```python
from build123d import *

# Parameters (mm, degrees)
F0_W          = 40
F0_H          = 25
F1_DEPTH      = 45
F2_R          = 5
F3_DEPTH      = 7
F4_R          = 2.5
F5_DEPTH      = 45.001
F5_DEPTH_BACK = 7.001
F6_R          = 2.5
F7_DEPTH      = 25.001


with BuildPart() as f1:
    # F0 (on Front) → F1 (new body)
    with BuildSketch(Plane.XZ):
        with Locations((-10, 0)):
            Rectangle(F0_W, F0_H)
    extrude(amount=-F1_DEPTH)

    # F2 (on face) → F3 (join)
    with BuildSketch(Plane.XZ):
        Circle(F2_R)
    extrude(amount=F3_DEPTH)

    # F4 (on Front) → F5 (cut, two sides)
    with BuildSketch(Plane.XZ) as f5_sk:
        Circle(F4_R)
    extrude(amount=-F5_DEPTH, mode=Mode.SUBTRACT)
    extrude(f5_sk.sketch, amount=F5_DEPTH_BACK, mode=Mode.SUBTRACT)

    # F6 (on face) → F7 (cut, through all)
    with BuildSketch(Plane.XY.offset(12.5)):
        with Locations((0, 21)):
            Circle(F6_R)
        with Locations((-10, 31)):
            Circle(F6_R)
        with Locations((-20, 21)):
            Circle(F6_R)
    extrude(amount=-F7_DEPTH, mode=Mode.SUBTRACT)


solid = f1.part
```
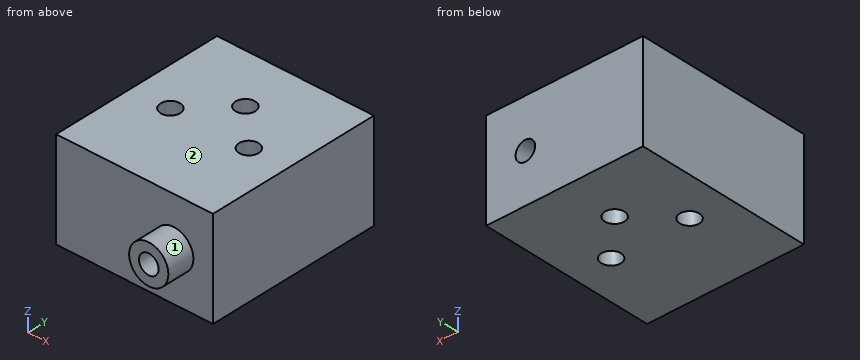
Geometry: final body of the model. Coordinates: model frame, mm. Face numbers are marked on the shaded views. A direction names the side the tool comes from. Coordinates: 2 decimals unless noted, no trailing zeros. Order: outer loops, then holes, each group sorted by start corner. A loop starts at its lowest first (then second) coordinate and runs counter-clockwise, first axis right, second up.
Item 1: Section query C-C (x = -10). Output: boundary loops of the cut face in (y, z), then the cut area to 3 significant figures.
Answer:
outline: (0, -12.5) - (28.5, -12.5) - (28.5, 12.5) - (0, 12.5) - close; (33.5, -12.5) - (45, -12.5) - (45, 12.5) - (33.5, 12.5) - close
area: 1,000 mm2
Item 2: Section query D-D (y = -1). Output: boundary loops of the cut face in (x, z), then the cut area to 3 significant figures.
Answer:
outline: circle Ø10 at (0, 0); hole circle Ø5 at (0, 0)
area: 58.9 mm2
Item 3: Section query A-A (x = 0). Output: boundary loops of the cut face in (y, z).
Answer:
outline: (-7, -5) - (0, -5) - (0, -12.5) - (18.5, -12.5) - (18.5, -2.5) - (-7, -2.5) - close; (-7, 2.5) - (18.5, 2.5) - (18.5, 12.5) - (0, 12.5) - (0, 5) - (-7, 5) - close; (23.5, -12.5) - (45, -12.5) - (45, -2.5) - (23.5, -2.5) - close; (23.5, 2.5) - (45, 2.5) - (45, 12.5) - (23.5, 12.5) - close
Item 4: Material intervals for line 1 along Y through (x, z) = (0, 4.75); line 2 along X through (y, z) = (14.5, 0); line 3 along Y through (x, z) = (-24, -9), sorted ascending.
Answer:
line 1: y = -7 to 18.5, 23.5 to 45
line 2: x = -30 to -2.5, 2.5 to 10
line 3: y = 0 to 45
Item 5: Section query B-B (z = 8). Output: boundary loops of the cut face in (x, y), then the cut area to 3 significant figures.
Answer:
outline: (-30, 0) - (10, 0) - (10, 45) - (-30, 45) - close; hole circle Ø5 at (-20, 21); hole circle Ø5 at (-10, 31); hole circle Ø5 at (0, 21)
area: 1,740 mm2
Item 6: Contact query for flat-ended pins moving along their axis: P1, Ø4, axis at x = 0, y = 21, coming from the +Z side; P2, Ø1.5, axis at x = -18.5, z = 0, coming from the -Y side; P3, Ø8, axis at x = -20, y = 21, coming from the +Z side. Output: stop coordinate, or through.
Answer:
P1: passes through
P2: stops at y = 0
P3: stops at z = 12.5
Item 7: Access query for the marked faces 1 and 2. Directions: +Z, -Z, +X, -X, +Y, -Y. A direction counts if a zero-diameter tool reaches every point of the face in a straight line with its end or side. Return the directions, or none.
Answer:
face 1: -Y
face 2: +Z, +X, -X, +Y, -Y
